Could you check a few things on this model? Use its own coordinates, in mm. Face numbers are marked on the shaded views. A direction names the side the tool comes from. Round coordinates to 2 decimals unless told otherwise and drop trailing zeros. Write each loop counter-clockwise with the first axis right and the second up, starting at its lowest first coordinate (ties: lowest second). Pieces come first, ordered by that corner, then holes. Notation, with made-up numbers: (67.5, 57) -> (95.5, 57) arc R18 cw to (95.5, 87) -> close; hole circle Ø4 at (-40, 42.25). An arc over 180 degrees is marked (long way). Answer in a Markdown table with one row per item. Add a question column.
```python
from build123d import *

# Parameters (mm, degrees)
SKETCH3_W           = 89
SKETCH3_H           = 44
BOSS_EXTRUDE1_DEPTH = 40
SKETCH4_R           = 20
BOSS_EXTRUDE2_DEPTH = 70
SKETCH5_R           = 4
BOSS_EXTRUDE3_DEPTH = 20


with BuildPart() as part:
    # Sketch3 → Boss-Extrude1 (new body)
    with BuildSketch(Plane(origin=(0, 0, 0), x_dir=(1, 0, 0), z_dir=(0, 1, 0))):
        Rectangle(SKETCH3_W, SKETCH3_H)
    extrude(amount=BOSS_EXTRUDE1_DEPTH)

    # Sketch4 → Boss-Extrude2 (add)
    with BuildSketch(Plane(origin=(0, 40, 0), x_dir=(1, 0, 0), z_dir=(0, 1, 0))):
        with Locations((22.662485516, 0)):
            Circle(SKETCH4_R)
    extrude(amount=BOSS_EXTRUDE2_DEPTH)

    # Sketch5 → Boss-Extrude3 (add)
    with BuildSketch(Plane(origin=(0, 40, 0), x_dir=(1, 0, 0), z_dir=(0, 1, 0))):
        with Locations((-39.5, -11)):
            Circle(SKETCH5_R)
        with Locations((-39.5, 11)):
            Circle(SKETCH5_R)
    extrude(amount=BOSS_EXTRUDE3_DEPTH)


solid = part.part
```
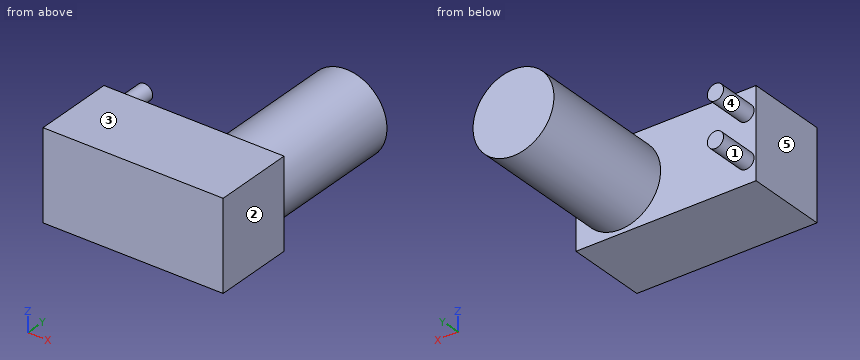
(1) Suppose I cut it at B-B, the plane z = -11. Please give me the cut outline in (x, y), then the cut area to 3 significant figures.
(2) Suppose I cut it at C-C, the plane y = 52. Please give me the cut outline in (x, z), then the cut area to 3 significant figures.
(3) On a 3-axis mill with a long thin cutter (end or side, diameter ignored), from which of +Z, -Z, +X, -X, +Y, -Y can I reach the whole of each face in a straight line? I mean the marked faces 1 and 2. Say none if no direction works.
(4) I need wall thicknesses on L1, parallel to Y at x = -30, z = -3.5; L2, parallel to X at y = 54.5, z = 8; L3, parallel to X at y = 52, z = 12. Which ranges of each line are inside material? Lowest first, please.
(5) For P1, Ø6.5, axis at x = -39.5, z = -12.5, coming from the +Y side; P2, Ø5, axis at y = 87.5, z = 5, coming from the +X side; P3, Ø1, axis at y = 52.5, z = -9.5, coming from the -X side, each with a flat end and sliding along its axis, tell me the tip position at first contact or that it passes through.
(6) Suppose I cut it at D-D, the plane y = 82. Please give me the cut outline in (x, z), then the cut area to 3 significant figures.
(7) If we mould it in two halves opening along X, with no side actions, what happens to the marked faces 3, 4 and 5? For each: pulls with the +X half, pulls with the -X half, needs draft (parallel to the pull), parting line crosses it, or undercut.
(8) Suppose I cut it at A-A, the plane x = -39.5. Please give me the cut outline in (y, z).
Response:
| question | item | result |
|---|---|---|
| 1 | outline | (-44.5, 0) -> (44.5, 0) -> (44.5, 40) -> (39.37, 40) -> (39.37, 110) -> (5.96, 110) -> (5.96, 40) -> (-35.5, 40) -> (-35.5, 60) -> (-43.5, 60) -> (-43.5, 40) -> (-44.5, 40) -> close |
| 1 | area | 6,060 mm² |
| 2 | outline | circle Ø8 at (-39.5, -11); circle Ø8 at (-39.5, 11); circle Ø40 at (22.66, 0) |
| 2 | area | 1,360 mm² |
| 3 | face 1 | +Y |
| 3 | face 2 | +Z, -Z, +X, +Y, -Y |
| 4 | L1 | 0 to 40 |
| 4 | L2 | -42.15 to -36.85, 4.33 to 40.99 |
| 4 | L3 | -43.37 to -35.63, 6.66 to 38.66 |
| 5 | P1 | y = 60 |
| 5 | P2 | x = 42.51 |
| 5 | P3 | x = -43.37 |
| 6 | outline | circle Ø40 at (22.66, 0) |
| 6 | area | 1,260 mm² |
| 7 | face 3 | needs draft |
| 7 | face 4 | undercut |
| 7 | face 5 | pulls with the -X half |
| 8 | outline | (0, -22) -> (40, -22) -> (40, -15) -> (60, -15) -> (60, -7) -> (40, -7) -> (40, 7) -> (60, 7) -> (60, 15) -> (40, 15) -> (40, 22) -> (0, 22) -> close |
